```python
from build123d import *

# Parameters (mm, degrees)
SKETCH2_R           = 2.75
SKETCH1_R           = 3.75
SKETCH3_R           = 2.45
SKETCH3_R_2         = 1.65
BOSS_EXTRUDE1_DEPTH = 1.7
BOSS_EXTRUDE2_START = 2
SKETCH4_R           = 3.25
SKETCH4_R_2         = 2.45
BOSS_EXTRUDE2_DEPTH = 2
SKETCH5_R           = 1.65
CUT_EXTRUDE1_DEPTH  = 11.880027642


with BuildPart() as part:
    # Sketch2 → Loft1 section 0
    with BuildSketch(Plane(origin=(0, 7.5, 0), x_dir=(1, 0, 0), z_dir=(0, 1, 0))):
        Circle(SKETCH2_R)
    # Sketch1 → Loft1 section 1
    with BuildSketch(Plane(origin=(0, 0, 0), x_dir=(1, 0, 0), z_dir=(0, 1, 0))):
        Circle(SKETCH1_R)
    loft()

    # Sketch3 → Boss-Extrude1 (add)
    with BuildSketch(Plane(origin=(0, 7.5, 0), x_dir=(1, 0, 0), z_dir=(0, 1, 0))):
        with Locations(Location((0, 0, 0), (0, 0, 270))):
            Circle(SKETCH3_R)
        with Locations(Location((0, 0, 0), (0, 0, 270))):
            Circle(SKETCH3_R_2, mode=Mode.SUBTRACT)
    extrude(amount=BOSS_EXTRUDE1_DEPTH)

    # Sketch4 → Boss-Extrude2 (add)
    with BuildSketch(Plane.XZ.offset(BOSS_EXTRUDE2_START)):
        with Locations(Location((0, 0, 0), (0, 0, 90))):
            Circle(SKETCH4_R)
        with Locations(Location((0, 0, 0), (0, 0, 90))):
            Circle(SKETCH4_R_2, mode=Mode.SUBTRACT)
    extrude(amount=-BOSS_EXTRUDE2_DEPTH)

    # Sketch5 → Cut-Extrude1 (cut, through all)
    with BuildSketch(Plane(origin=(0, 7.5, 0), x_dir=(1, 0, 0), z_dir=(0, 1, 0))):
        with Locations(Location((0, 0, 0), (0, 0, 270))):
            Circle(SKETCH5_R)
    extrude(amount=-CUT_EXTRUDE1_DEPTH, mode=Mode.SUBTRACT)


solid = part.part
```
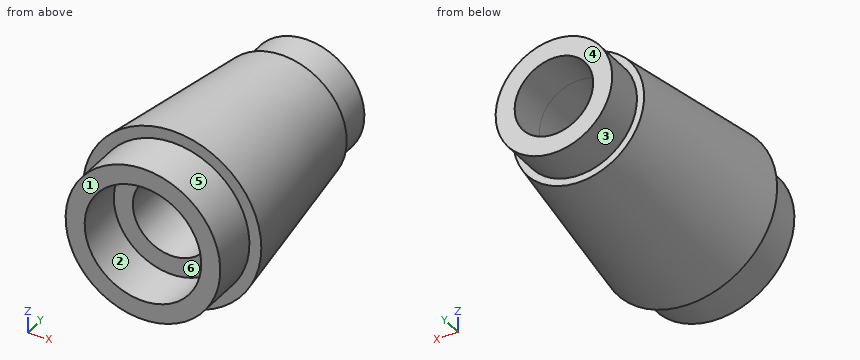
The listing builds one solid part. Answer for the finished solid, in the listing's coordinates (mm). Face numbers are marked on the shaded views. A direction names the side the tool comes from. Give positions to 0.01 mm unless a question says otherwise; leave off trailing zeros. Order: outer loops, then holes, each group sorted by start corner. A loop starts at its lowest first (then second) coordinate and runs counter-clockwise, first axis right, second up. Notation, with made-up numbers: (80.25, 11.5) -> (114.25, 11.5) arc R20 ccw to (114.25, 27.5) -> close; hole circle Ø6 at (59.5, 73.25). An arc over 180 degrees is marked (long way). Answer as a JSON object with one key per item and string values. Group by question number.
Item 1: The part is cut by section A-A on x = 0. Write down the section's boundary in (y, z).
Item 2: The part is cut by section B-B on y = -1. Write down the section's boundary in (x, z), and give its area (3 significant figures).
Item 3: Consider L1, parallel to X at y = -1.4, z = 0; L2, parallel to Z at x = -0.5, y = 6.25; L3, parallel to X at y = 8.25, z = 0. Determine where each line is inside the solid, lowest interval first. Write a range as from..to.
Item 4: A tool of negligible diameter and unlimited length cuts with its end or side. For the marked faces 1, 2 and 3, from which of +Z, -Z, +X, -X, +Y, -Y can it reach the whole face along a straight path? Write none if from no direction.
Item 5: Determine the mould class of the marked faces 4, 5 and 6 for opening direction Z: pulls with the +Z half, pulls with the -Z half, needs draft (parallel to the pull), parting line crosses it, or undercut.
Item 6: The part is cut by section C-C on y = 7.75. Write down the section's boundary in (x, z), and give its area (3 significant figures).
Item 7: Flat-ended cylindrical pins translate along their axes: pin 1 (1 mm diameter, centred on x = 1, y = 2.5, fed in from +Z); pin 2 (3 mm diameter, centred on y = 3.5, z = -0.5, fed in from +X); pin 3 (1.5 mm diameter, centred on y = 3.5, z = -1.5, fed in from -X); pin 4 (3 mm diameter, centred on x = 0, z = 0, fed in from -Y). Find the tip coordinate at first contact, or state that the pin passes through.
Result set:
{
 "1": {"outline": "(-2, -3.25) -> (0, -3.25) -> (0, -3.75) -> (7.5, -2.75) -> (7.5, -2.45) -> (9.2, -2.45) -> (9.2, -1.65) -> (0, -1.65) -> (0, -2.45) -> (-2, -2.45) -> close; (-2, 2.45) -> (0, 2.45) -> (0, 1.65) -> (9.2, 1.65) -> (9.2, 2.45) -> (7.5, 2.45) -> (7.5, 2.75) -> (0, 3.75) -> (0, 3.25) -> (-2, 3.25) -> close"},
 "2": {"outline": "circle Ø6.5 at (0, 0); hole circle Ø4.9 at (0, 0)", "area": "14.3 mm²"},
 "3": {"L1": "-3.25..-2.45, 2.45..3.25", "L2": "-2.87..-1.57, 1.57..2.87", "L3": "-2.45..-1.65, 1.65..2.45"},
 "4": {"face 1": "+Z, -Z, +X, -X, -Y", "face 2": "-Y", "face 3": "+Y"},
 "5": {"face 4": "needs draft", "face 5": "parting line crosses it", "face 6": "undercut"},
 "6": {"outline": "circle Ø4.9 at (0, 0); hole circle Ø3.3 at (0, 0)", "area": "10.3 mm²"},
 "7": {"pin 1": "z = 3.4", "pin 2": "x = 3.47", "pin 3": "x = -3.22", "pin 4": "through"}
}
